Autodesk Inventor part; units mm, degrees
ref_plane "Work Plane1" through (0, 0, -7.5) normal (0, 0, -1) x (-1, 0, 0)
ref_plane "YZ Plane" through (0, 0, 0) normal (1, 0, 0) x (0, 1, 0)
ref_plane "XZ Plane" through (0, 0, 0) normal (0, 1, 0) x (-1, 0, 0)
sketch "Sketch1" plane through (0, 0, 0) normal (1, 0, 0) x (0, 1, 0)
  circle A0 centre (0, 0) radius 6
  line L0 (0, 6) -> (0, -6)
  line L1 (3, -5.1962) -> (3, 5.1962)
  line L2 (3.9686, 4.5) -> (3, 4.5)
  line L3 (3.9686, -4.5) -> (3, -4.5)
  dimension "d0" = 6
  dimension "d1" = 9
  dimension "d2" = 12
revolve "Revolution1" add sketch "Sketch1" angle 360 about axis through (0, 0, 6) along (0, 0, -1) contours A0 L3 L1 L2
sketch "Sketch2" plane through (0, 0, 4.5) normal (0, 0, 1) x (1, 0, 0)
  circle A0 centre (0, 0) radius 3
  dimension "d4" = 6
extrude "Extrusion1" add sketch "Sketch2" against normal blind 29
ref_plane "Work Plane1" through (0, 0, -7.5) normal (0, 0, -1) x (-1, 0, 0)
sketch "Sketch3" plane through (0, 0, -7.5) normal (0, 0, -1) x (-1, 0, 0)
  line L0 (4, -2.3094) -> (0, -4.6188)
  line L1 (0, -4.6188) -> (-4, -2.3094)
  line L2 (-4, -2.3094) -> (-4, 2.3094)
  line L3 (-4, 2.3094) -> (0, 4.6188)
  line L4 (0, 4.6188) -> (4, 2.3094)
  line L5 (4, 2.3094) -> (4, -2.3094)
  point P0 (0, 0)
  point P1 (0, 0)
  dimension "d8" = 8
extrude "Extrusion2" add sketch "Sketch3" along normal blind 3
chamfer "Chamfer1" distance 1 angle 45 1 edges at (-3, 0, -24.5)
thread "Thread1"
properties part number "Ball" material "Steel, Carbon"
Input: part model. Units: mm. Frame: model coordinates. A direction names the side the tool comes from. Round coordinates to 2 decimals unless told otherwise and drop trailing zeros. Loops run counter-clockwise (first coordinate to the right, second up) from the corner with the lowest first, then second, coordinate; pieces in that order, holes last. Notation, with made-up numbers: M -8,50.25 L 0,50.25 A31 cw 0,79.25 Z; hole C 61.5,8.25 d9. An arc over 180 degrees is marked long. Answer in a Markdown table with one row per item. Add a question column.
1. Section C-C (z = -2.5). Output: boundary loops of the cut face in (x, y).
2. Mould query, pull axis Z, two halves, no side actions, for faces 1 (the face through (1, -3, -10.5)), 2 (the face through (4, 0, -9)), 3 (the face through (1, -3, -7.5)), 4 (the face through (3, 1, -4.5)). Classes: released by +Z, released by -Z, zero draft, split by the parting line, or undercut.
3. Section A-A (z = -20). Output: boundary loops of the cut face in (x, y), and give its area (3 significant figures).
4. Ray query, probe 1 along Z at (x, y) = (0, 4.5); probe 2 along Z at (x, y) = (-2.5, -2.25); probe 3 along X at (y, z) = (-1.25, 2). Return the intervals inside material, ascending.
5. Set-up query: faces 5 (the face through (-4, 0, -9)), 6 (the face through (-3, 0, -17)), 7 (the face through (-1.97, 3.48, -8.98)), 8 (the face through (1.97, -3.48, -8.98)), 9 (the face through (-2.028, -3.448, -8.979)). Return all of +Z, -Z, +X, -X, +Y, -Y with unobstructed straight access to the full face (end or side cutting, diameter ignored); none if empty.
6. Contact query for flat-ended pins moving along their axis: pin 1 (5 mm diameter, centred on x = -4, z = -17, fed in from +Y); pin 2 (1.5 mm diameter, centred on x = -0.5, z = 1, fed in from +Y); pin 3 (2.5 mm diameter, centred on y = 0, z = -9.5, fed in from +X); pin 4 (2.5 mm diameter, centred on x = -2, y = 0.5, fed in from -Z). Output: stop coordinate, or through.
7. Section B-B (y = 0). Output: boundary loops of the cut face in (x, z).
Values follow:
| question | item | result |
|---|---|---|
| 1 | outline | C 0,0 d10.91 |
| 2 | face 1 | released by -Z |
| 2 | face 2 | zero draft |
| 2 | face 3 | undercut |
| 2 | face 4 | undercut |
| 3 | outline | C 0,0 d6 |
| 3 | area | 28.3 mm^2 |
| 4 | probe 1 | -10.5 to -7.5, -3.97 to 3.97 |
| 4 | probe 2 | -10.5 to -7.5, -4.5 to 4.5 |
| 4 | probe 3 | -5.52 to 5.52 |
| 5 | face 5 | -Z, -X, +Y, -Y |
| 5 | face 6 | -Z |
| 5 | face 7 | -Z, -X, +Y |
| 5 | face 8 | -Z, +X, -Y |
| 5 | face 9 | -Z, -X, -Y |
| 6 | pin 1 | y = 2.6 |
| 6 | pin 2 | y = 5.99 |
| 6 | pin 3 | x = 4 |
| 6 | pin 4 | z = -24.5 |
| 7 | outline | M -4,-10.5 L -3,-10.5 L -3,-23.5 L -2,-24.5 L 2,-24.5 L 3,-23.5 L 3,-10.5 L 4,-10.5 L 4,-7.5 L 3,-7.5 L 3,-4.5 L 3.97,-4.5 A6 ccw 3.97,4.5 L -3.97,4.5 A6 ccw -3.97,-4.5 L -3,-4.5 L -3,-7.5 L -4,-7.5 Z |
